Work out the finished part from the listing and answer in its coordinate system (mm). A direction names the side the tool comes from. Coordinates: 2 decimals unless noted, no trailing zeros. Write each loop counter-clockwise with the first axis right and the second up, starting at its lowest first coordinate (ties: lowest second). Pieces come first, ordered by that corner, then holes. Notation, with made-up numbers: (79.25, -11) - (102.25, -11) arc R17 cw to (102.25, 18) - close; hole circle Ø10 at (69.25, 3.25). An arc over 180 degrees is marked (long way). Use a Markdown table: item, result. Add a question column.
(1) The part is cut by section C-C, the plane y = -52.5. Give the vertices of the cut face in (x, z), then the cut area to 3 significant figures.
(2) The part is cut by section A-A, the plane x = 42. Give the vertices of the cut face in (y, z).
(3) For a pull along Y with two mould halves and no side action, classify faces 3 (the face through (-1, -110.49, 1)), 4 (the face through (-5, -112, -50.8)), 5 (the face through (-1, 0, 1)), 6 (the face through (-1, -114.3, 1)) as released by +Y, released by -Y, zero draft, split by the parting line, or undercut.
(4) Given pin 1 Ø12 at (x, y) = (-36, -98.5) entering from -Z, flat-ended and moving along its own axis, determine where the tip first touches the part or whether it passes through.
(5) A tool of negligible diameter and unlimited length cuts with its end or side. For faces 1 (the face through (-57.15, -56, -1)), 2 (the face through (53.34, -58, 1)), from which of +Z, -Z, +X, -X, +Y, -Y can it reach the whole face along a straight path? Write none if from no direction.
(6) The part is cut by section B-B, the plane z = -16. Give the vertices of the cut face in (x, y), then the cut area to 3 significant figures.
(7) Find the intervals of material crossed by line 1 (Y direction, x = 37, z = 45); line 2 (X direction, y = -85.5, z = -24.5), in increasing order. Write a range as from..to.
from build123d import *

# Parameters (mm, degrees)
F0_W     = 114.3
F0_H     = 101.6
F1_DEPTH = 114.3
F2_W     = 106.68
F2_H     = 106.68
F3_DEPTH = 50.801
F4_DEPTH = 50.801


with BuildPart() as f1:
    # F0 (on Front) → F1 (new body)
    with BuildSketch(Plane.XZ):
        Rectangle(F0_W, F0_H)
    extrude(amount=F1_DEPTH)

    # F2 (on Top) → F3 (cut, through all)
    with BuildSketch(Plane.XY):
        with Locations((0, -57.15)):
            Rectangle(F2_W, F2_H)
    extrude(amount=F3_DEPTH, mode=Mode.SUBTRACT)

    # F2 (on Top) → F4 (cut, through all)
    with BuildSketch(Plane.XY):
        with Locations((0, -57.15)):
            Rectangle(F2_W, F2_H)
    extrude(amount=-F4_DEPTH, mode=Mode.SUBTRACT)


solid = f1.part
Model answer:
| question | item | result |
|---|---|---|
| 1 | outline | (-57.15, -50.8) - (-53.34, -50.8) - (-53.34, 50.8) - (-57.15, 50.8) - close; (53.34, -50.8) - (57.15, -50.8) - (57.15, 50.8) - (53.34, 50.8) - close |
| 1 | area | 774 mm^2 |
| 2 | outline | (-114.3, -50.8) - (-110.49, -50.8) - (-110.49, 50.8) - (-114.3, 50.8) - close; (-3.81, -50.8) - (0, -50.8) - (0, 50.8) - (-3.81, 50.8) - close |
| 3 | face 3 | undercut |
| 3 | face 4 | zero draft |
| 3 | face 5 | released by +Y |
| 3 | face 6 | released by -Y |
| 4 | pin 1 | through |
| 5 | face 1 | +Z, -Z, -X, +Y, -Y |
| 5 | face 2 | +Z, -Z |
| 6 | outline | (-57.15, -114.3) - (57.15, -114.3) - (57.15, 0) - (-57.15, 0) - close; hole (-53.34, -110.49) - (53.34, -110.49) - (53.34, -3.81) - (-53.34, -3.81) - close |
| 6 | area | 1,680 mm^2 |
| 7 | line 1 | -114.3..-110.49, -3.81..0 |
| 7 | line 2 | -57.15..-53.34, 53.34..57.15 |
